from build123d import *

# Parameters (mm, degrees)
SKETCH1_W           = 24
SKETCH1_H           = 24
BOSS_EXTRUDE1_DEPTH = 1.5
CHAMFER1_SIZE       = 1
SKETCH2_R           = 1
CUT_EXTRUDE1_DEPTH  = 1.5


with BuildPart() as part:
    # Sketch1 → Boss-Extrude1 (new body)
    with BuildSketch(Plane(origin=(0, 0, 0), x_dir=(1, 0, 0), z_dir=(0, 1, 0))):
        Rectangle(SKETCH1_W, SKETCH1_H)
    extrude(amount=BOSS_EXTRUDE1_DEPTH)

    # Chamfer1
    chamfer1_edges = [part.edges().sort_by_distance(p)[0] for p in [
        (-12, 0.75, -12),
        (12, 0.75, -12),
        (12, 0.75, 12),
        (-12, 0.75, 12),
    ]]
    chamfer(chamfer1_edges, length=CHAMFER1_SIZE)

    # Sketch2 → Cut-Extrude1 (cut)
    with BuildSketch(Plane(origin=(0, 1.5, 0), x_dir=(1, 0, 0), z_dir=(0, 1, 0))):
        with Locations(Location((-10, 10, 0), (0, 0, 270))):
            Circle(SKETCH2_R)
        with Locations(Location((10, 10, 0), (0, 0, 270))):
            Circle(SKETCH2_R)
        with Locations(Location((10, -10, 0), (0, 0, 270))):
            Circle(SKETCH2_R)
        with Locations(Location((-10, -10, 0), (0, 0, 270))):
            Circle(SKETCH2_R)
    extrude(amount=-CUT_EXTRUDE1_DEPTH, mode=Mode.SUBTRACT)


solid = part.part
Work out the finished part from the listing and answer in its coordinate system (mm). Round coordinates to 2 decimals unless told otherwise and drop trailing zeros. Write each loop counter-clockwise with the first axis right and the second up, starting at its lowest first coordinate (ties: lowest second). Pieces come first, ordered by that corner, then holes. Notation, with made-up numbers: (20.25, -19) - (68.25, -19) arc R24 cw to (68.25, -6) - close; hole circle Ø9 at (16, 73.25). An arc over 180 degrees is marked (long way). Answer in a Markdown table with one row per item. Add a question column.
1. Find the intervals of material crossed by line 1 along X through (y, z) = (0.45, 10); line 2 along Z through (x, y) = (10.5, 0.65), in increasing order. Write a range as from..to.
2. A cutting plane is placed at A-A, the plane z = -10. Determine the outline of the cut face in (x, y), and give its area (3 significant figures).
3. A cutting plane is placed at B-B, the plane x = -10. Determine the outline of the cut face in (y, z), and give its area (3 significant figures).
4. The mould has two halves that part along X. Classify faces 1 (the flat face through (11.5, 0.7, 11.5)), 2 (the flat face through (0, 0, 0)), 3 (the cylindrical face through (11, 1, 10)): +X half, -X half, draft (parallel to the pull), parting line (faces both ways), or undercut.
Worked out:
| question | item | result |
|---|---|---|
| 1 | line 1 | -12..-11, -9..9, 11..12 |
| 1 | line 2 | -12..-10.87, -9.13..9.13, 10.87..12 |
| 2 | outline | (-12, 0) - (-11, 0) - (-11, 1.5) - (-12, 1.5) - close; (-9, 0) - (9, 0) - (9, 1.5) - (-9, 1.5) - close; (11, 0) - (12, 0) - (12, 1.5) - (11, 1.5) - close |
| 2 | area | 30.0 mm^2 |
| 3 | outline | (0, -12) - (1.5, -12) - (1.5, -11) - (0, -11) - close; (0, -9) - (1.5, -9) - (1.5, 9) - (0, 9) - close; (0, 11) - (1.5, 11) - (1.5, 12) - (0, 12) - close |
| 3 | area | 30.0 mm^2 |
| 4 | face 1 | +X half |
| 4 | face 2 | draft |
| 4 | face 3 | undercut |
